Build history of the part. All positions in model axes, mm. A direction names the side the tool comes from. Round coordinates to 2 decimals unless told otherwise and drop trailing zeros. Write each loop counter-clockwise with the first axis right and the second up, starting at its lowest first coordinate (ties: lowest second). Pieces come first, ordered by that corner, then holes. Notation, with made-up numbers: (79.5, -7.75) -> (135.5, -7.75) arc R26 cw to (135.5, 6.25) -> close; hole circle Ø6 at (22, 57). An arc over 180 degrees is marked (long way). Answer in a Markdown table with one row per item. Add a question column.
Autodesk Inventor part; units mm, degrees
ref_plane "YZ Plane" through (0, 0, 0) normal (1, 0, 0) x (0, 1, 0)
ref_plane "XZ Plane" through (0, 0, 0) normal (0, 1, 0) x (-1, 0, 0)
ref_plane "XY Plane" through (0, 0, 0) normal (0, 0, 1) x (1, 0, 0)
sketch "Sketch1" plane through (0, 0, 0) normal (1, 0, 0) x (0, 1, 0)
  line L0 (-191.1, 0) -> (191.1, 0) construction
  line L1 (0, -46) -> (0, 66) construction
  line L2 (-136.5, 30) -> (136.5, 30)
  line L3 (136.5, 30) -> (136.5, -30)
  line L4 (136.5, -30) -> (-136.5, -30)
  line L5 (-136.5, -30) -> (-136.5, 30)
  line L6 (105.4423, 30) -> (136.5, 50)
  line L7 (136.5, 50) -> (136.5, 30)
  circle A0 centre (133.5, 44.4999) radius 3
  circle A1 centre (115.5, 32.9086) radius 3
  line L8 (-136.5, 30) -> (103.5, 30) construction
  line L9 (103.5, 30) -> (103.5, 38) construction
  line L10 (103.5, 38) -> (-136.5, 38) construction
  line L11 (-136.5, 38) -> (-136.5, 30) construction
  line L12 (112.5, 34.5449) -> (112.5, 30)
  circle A2 centre (109.5, 30) radius 3
  circle A3 centre (109.5, 33) radius 3
  line L13 (-56.5, 30) -> (3.5, 30)
  line L14 (3.5, 30) -> (3.5, 0)
  line L15 (3.5, 0) -> (-56.5, 0)
  line L16 (-56.5, 0) -> (-56.5, 30)
  line L17 (-26.5, 0) -> (-26.5, 30) construction
  point P0 (0, 0)
  point P1 (106.5, 30)
  dimension "d6" = 6
  dimension "d1" = 32.78
  dimension "d2" = 6
  dimension "d3" = 8
  dimension "d4" = 240
  dimension "d7" = 60
  dimension "d35" = 147.22
  dimension "d36" = 273
  dimension "d37" = 20
  dimension "d38" = 24
  dimension "d39" = 110
  dimension "d40" = 60
  dimension "d41" = 30
extrude "Extrusion1" add sketch "Sketch1" along normal mid plane 10 contours L2 L16 L15 L14 A2 A1 L3 L4 L5 | L2 L14 L15 L16 | L2 A2 | A1 L2 picked at (115.4176, 29.9729)
extrude "Extrusion2" cut sketch "Sketch1" along normal through all both and the other way through all contours L2 L14 L15 L16
sketch "Sketch2" plane through (-5, -136.5, 30) normal (0, 0, 1) x (1, 0, 0)
  line L0 (5, -54.6) -> (5, 327.6) construction
  line L1 (0, 0) -> (10, 0)
  point P0 (5, 136.5)
  point P1 (5, 72.5)
  point P2 (5, 147.5)
  point P3 (5, 222.5)
  dimension "d11" = 72.5
  dimension "d12" = 75
  dimension "d13" = 75
hole "Hole1" at (0, -64, 30) at (0, 11, 30) at (0, 86, 30) direction (0, 0, -1) diameter 3.242 depth 15 tip angle 118
sketch "Sketch3" plane through (5, 136.5, -30) normal (0, 0, -1) x (-1, 0, 0)
  line L0 (12, -136.5) -> (-2, -136.5) construction
  line L1 (5, -327.6) -> (5, 54.6) construction
  point P0 (5, -136.5)
  point P1 (5, -261.5)
  point P2 (5, -136.5)
  point P3 (5, -11.5)
  dimension "d21" = 250
hole "Hole2" at (0, -125, -30) at (0, 0, -30) at (0, 125, -30) direction (0, 0, 1) diameter 3.242 depth 15 tip angle 118
fillet "Fillet1" radius 3 2 edges at (0, -56.5, 0) (0, 3.5, 0)
fillet "Fillet1" radius 1 4 edges at (0, -56.5, 30) (0, 3.5, 30) (0, -136.5, 30) (0, 136.5, 30)
properties part number "GRJ-04-103" material "Fenolite OR"
(1) Drop flat-ended pins along their axis: P1, Ø1.9, axis at x = 0, y = -125, coming from the -Z side; P2, Ø5, axis at x = -0.5, y = -24, coming from the +Z side. Give the stop position or say it passes through.
(2) Saw through at B-B (y = -25). List the corners of the cut face in (x, z), plus the area to 3 significant figures.
(3) Probe line 1 along Y through (x, z) = (0, 25.5); line 2 along X through (y, z) = (11, 26.75); line 3 along Y through (x, z) = (1, 10). List the from-to ranges inside material, lowest first.
(4) Which spindle directions (+Z, -Z, +X, -X, +Y, -Y) get a long thin tool onto all of the face, cutting with end or side? Do faces 5 (the face through (-5, -2, -6)), 6 (the face through (0, 3.5, 16)). Say none if no direction does.
(5) Mould opens along Y. For faces 1 (the face through (0, -97, 30)), 2 (the face through (0, 136.5, 0)), 3 (the face through (0, -26, 0)), 4 (the face through (0, -136.5, -1)) say: pulls with the +Y half, pulls with the -Y half, needs draft (parallel to the pull), parting line crosses it, or undercut.
(6) Saw through at A-A (x = 3.5). List the corners of the cut face in (y, z), plus the area to 3 significant figures.
Answer sheet:
| question | item | result |
|---|---|---|
| 1 | P1 | stops at z = -14.6 |
| 1 | P2 | stops at z = 0 |
| 2 | outline | (-5, -30) -> (5, -30) -> (5, 0) -> (-5, 0) -> close |
| 2 | area | 300 mm² |
| 3 | line 1 | y = -136.5 to -65.62, -62.38 to -56.5, 3.5 to 9.38, 12.62 to 84.38, 87.62 to 136.5 |
| 3 | line 2 | x = -5 to -1.62, 1.62 to 5 |
| 3 | line 3 | y = -136.5 to -56.5, 3.5 to 136.5 |
| 4 | face 5 | +Z, -Z, -X, +Y, -Y |
| 4 | face 6 | +Z, +X, -X |
| 5 | face 1 | needs draft |
| 5 | face 2 | pulls with the +Y half |
| 5 | face 3 | undercut |
| 5 | face 4 | pulls with the -Y half |
| 6 | outline | (-136.5, -30) -> (136.5, -30) -> (136.5, 29) arc R1 ccw to (135.5, 30) -> (4.5, 30) arc R1 ccw to (3.5, 29) -> (3.5, 3) arc R3 cw to (0.5, 0) -> (-53.5, 0) arc R3 cw to (-56.5, 3) -> (-56.5, 29) arc R1 ccw to (-57.5, 30) -> (-135.5, 30) arc R1 ccw to (-136.5, 29) -> close |
| 6 | area | 14,600 mm² |
